from build123d import *
from build123d import SkipClean  # not in build123d's __all__

# Parameters (mm, degrees)
F0_W     = 107.8271307051
F0_H     = 79.9957364798
F1_DEPTH = 69.342
F3_DEPTH = 171.704
F4_DEPTH = 25.4
F6_DEPTH = 25.4
F7_R     = 9.3550857854
F8_DEPTH = 220.218
F7_R_2   = 7.7300183475
F9_DEPTH = 194.31


# Not quite as in the source:
# - after a boolean that leaves OpenCascade's solid faulty, fix() repairs it


with BuildPart() as f1:
    # F0 (on Top) → F1 (new body)
    with BuildSketch(Plane.XY):
        with Locations((-0.6197858602, -6.3926763833)):
            Rectangle(F0_W, F0_H)
    extrude(amount=F1_DEPTH)

    # F2 (on face) → F3 (cut)
    with BuildSketch(Plane.XZ.offset(46.3905446231)):
        with BuildLine():
            Line((19.6710973978, 69.342), (-14.813689515, 69.342))
            ThreePointArc((-14.813689515, 69.342), (2.4287039414, 49.9755106866), (19.6710973978, 69.342))
        make_face()
    extrude(amount=-F3_DEPTH, mode=Mode.SUBTRACT)

    # F2 (on face) → F4 (join)
    with BuildSketch(Plane.XZ.offset(46.3905446231)):
        with BuildLine():
            Line((-14.813689515, 69.342), (-32.0560820401, 69.342))
            ThreePointArc((-32.0560820401, 69.342), (1.3510622084, 33.9996767093), (34.7582064569, 69.342))
            Line((34.7582064569, 69.342), (19.6710973978, 69.342))
            ThreePointArc((19.6710973978, 69.342), (2.4287039414, 49.9755106866), (-14.813689515, 69.342))
        make_face()
    with SkipClean():  # cleaning this boolean's faces spoils the solid; the shape is the same uncleaned
        extrude(amount=F4_DEPTH)

    # F5 (on face) → F6 (join)
    with BuildSketch(Plane(origin=(0, 33.6051918566, 0), x_dir=(-1, 0, 0), z_dir=(0, 1, 0))):
        with BuildLine():
            Line((-19.6710973978, 69.342), (-36.4824384451, 69.342))
            ThreePointArc((-36.4824384451, 69.342), (-0.9044590406, 35.2025825454), (34.6735203639, 69.342))
            Line((34.6735203639, 69.342), (14.813689515, 69.342))
            ThreePointArc((14.813689515, 69.342), (-2.4287039414, 49.9755106866), (-19.6710973978, 69.342))
        make_face()
    extrude(amount=F6_DEPTH)

    add(f1.part.fix(), mode=Mode.REPLACE)

    # F7 (on face) → F8 (cut)
    with BuildSketch(Plane.XY.offset(69.342)):
        with Locations((-35.963576287, -7.5180209242)):
            Circle(F7_R)
    extrude(amount=-F8_DEPTH, mode=Mode.SUBTRACT)

    # F7 (on face) → F9 (cut)
    with BuildSketch(Plane.XY.offset(69.342)):
        with Locations((42.4882248044, -6.3926763833)):
            Circle(F7_R_2)
    extrude(amount=-F9_DEPTH, mode=Mode.SUBTRACT)


solid = f1.part
Verification items for the finished model (mm, model axes). A direction names the side the tool comes from. Coordinates: 2 decimals unless noted, no trailing zeros. Order: outer loops, then holes, each group sorted by start corner. A loop starts at its lowest first (then second) coordinate and runs counter-clockwise, first axis right, second up.
1. Scan lines: line 1 (Y direction, x = -11.5, z = 31.5); line 2 (X direction, y = -5.5, z = 65); line 3 (Y direction, x = 47, z = 41). Record each from-to range of solid material in increasing order.
Results found:
line 1: y = -46.39 to 33.61
line 2: x = -54.53 to -45.1, -26.83 to -14.77, 19.63 to 34.81, 50.17 to 53.29
line 3: y = -46.39 to -12.67, -0.12 to 33.61
2. Sectioned sample at C-C, the plane y = -4.5. Record the cut outline in (x, z), and give its area (3 significant figures).
Results found:
outline: (-54.53, 0) - (-44.82, 0) - (-44.82, 69.34) - (-54.53, 69.34) - close; (-27.11, 0) - (34.99, 0) - (34.99, 69.34) - (19.67, 69.34) arc R17.36 cw (long way) to (-14.81, 69.34) - (-27.11, 69.34) - close; (49.98, 0) - (53.29, 0) - (53.29, 69.34) - (49.98, 69.34) - close
area: 4,670 mm2
3. Sectioned sample at A-A, the plane z = 54. Record the cut outline in (x, y), and give its area (3 significant figures).
Results found:
outline: (-54.53, -46.39) - (-29.28, -46.39) - (-29.28, -71.79) - (-8.69, -71.79) - (-8.69, 59.01) - (-30.49, 59.01) - (-30.49, 33.61) - (-54.53, 33.61) - close; (13.54, -71.79) - (31.98, -71.79) - (31.98, -46.39) - (53.29, -46.39) - (53.29, 33.61) - (32.29, 33.61) - (32.29, 59.01) - (13.54, 59.01) - close; hole circle Ø18.71 at (-35.96, -7.52); hole circle Ø15.46 at (42.49, -6.39)
area: 8,410 mm2
4. Sectioned sample at D-D, the plane z = 44. Record the cut outline in (x, y).
Results found:
outline: (-54.53, -46.39) - (-22.51, -46.39) - (-22.51, -71.79) - (25.21, -71.79) - (25.21, -46.39) - (53.29, -46.39) - (53.29, 33.61) - (24.34, 33.61) - (24.34, 59.01) - (-22.53, 59.01) - (-22.53, 33.61) - (-54.53, 33.61) - close; hole circle Ø18.71 at (-35.96, -7.52); hole circle Ø15.46 at (42.49, -6.39)
5. Release check for a two-part mould opening along X. For faces 1 (the face through (-45.31, -7.11, 35.16)), 2 (the face through (1, -59, 34)), 3 (the face through (49.86, -4.07, 35.16)), 4 (the face through (1, -71.791, 48)) record: +X half, -X half, draft (parallel to the pull), parting line (faces both ways), or undercut.
Results found:
face 1: undercut
face 2: parting line
face 3: undercut
face 4: draft
6. Sectioned sample at B-B, the plane x = -42. Record the cut outline in (y, z) (3 decimals).
Results found:
outline: (-46.391, 0) - (-14.665, 0) - (-14.665, 69.342) - (-46.391, 69.342) - close; (-0.371, 0) - (33.605, 0) - (33.605, 69.342) - (-0.371, 69.342) - close
7. Go/stop test with flat-tipped pins: pin 1 Ø6 at (x, z) = (0, 30) entering from -Y; pin 2 Ø21 at (x, z) = (2.43, 67.33) entering from -Y; pin 3 Ø2 at (x, y) = (17.5, 39.5) entering from -Z. Record where each tip stops, or that it passes through.
Results found:
pin 1: stops at y = -46.39
pin 2: passes through
pin 3: stops at z = 38.8
8. Set-up check for faces 5 (the face through (-1, -46.391, 26)), 6 (the face through (1, 59.005, 49)), 7 (the face through (1.67, 46.13, 35.21)): record each of +Z, -Z, +X, -X, +Y, -Y from which the full face is reachable in a straight line by a thin tool's end or side.
Results found:
face 5: -Z, -Y
face 6: +Z, -Z, +X, -X, +Y
face 7: -Z, +Y
